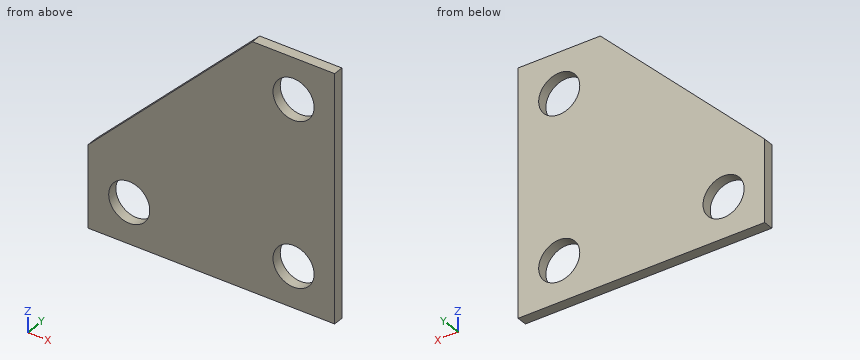
Autodesk Inventor part; units mm, degrees
ref_plane "YZ Plane" through (0, 0, 0) normal (1, 0, 0) x (0, 1, 0)
ref_plane "XZ Plane" through (0, 0, 0) normal (0, 1, 0) x (-1, 0, 0)
ref_plane "XY Plane" through (0, 0, 0) normal (0, 0, 1) x (1, 0, 0)
sketch "Sketch1" plane through (0, 0, 0) normal (0, 1, 0) x (-1, 0, 0)
  line L0 (0, 0) -> (76.2, 0)
  line L1 (76.2, 0) -> (76.2, 25.4)
  line L2 (25.4, 76.2) -> (0, 76.2)
  line L3 (0, 76.2) -> (0, 0)
  line L4 (76.2, 25.4) -> (25.4, 76.2)
  circle A0 centre (63.5, 12.7) radius 6.35
  circle A1 centre (12.7, 63.5) radius 6.35
  circle A2 centre (12.7, 12.7) radius 6.35
  point P0 (76.2, 76.2)
  dimension "d0" = 76.2
  dimension "d1" = 76.2
  dimension "d2" = 50.8
  dimension "d3" = 50.8
  dimension "d4" = 12.7
  dimension "d5" = 12.7
  dimension "d6" = 12.7
  dimension "d7" = 12.7
  dimension "d8" = 50.8
  dimension "d9" = 50.8
  dimension "d10" = 12.7
  dimension "d11" = 12.7
  dimension "d12" = 12.7
extrude "Extrusion1" add sketch "Sketch1" along normal blind 3.175
equation "\"d0\" = d1"
properties part number "3 inch gusset plate"
For this review, take the finished solid that the model builds, in its own axes (mm). Round coordinates to 2 decimals unless told otherwise and drop trailing zeros. Write each loop counter-clockwise with the first axis right and the second up, starting at its lowest first coordinate (ties: lowest second). Pieces come first, ordered by that corner, then holes. Notation, with made-up numbers: (-3.5, -34.75) - (21.5, -34.75) arc R23 ccw to (21.5, -1.75) - close; hole circle Ø1 at (4, 37.25). An arc over 180 degrees is marked (long way). Answer as CSV lines item,"result". Start each with the question number.
(1) Add section B-B, the plane y = 1.05. State the section outline as (x, z) points.
(2) Add section A-A, the plane z = 63.5. State the section outline as (x, y) points (3 decimals).
(3) Add section C-C, the plane x = -12.7. State the section outline as (y, z) points (3 decimals), plus the area to 3 significant figures.
(4) Add section D-D, the plane z = 12.7. State the section outline as (x, y) points (3 decimals), plus the area to 3 significant figures.
(5) For line 1 (Z direction, x = -12.7, y = 1.4); line 2 (Z direction, x = -18.5, y = 0.4); line 3 (X direction, y = 2.95, z = 7), list the stretches that pass through material, from the lowest coordinate up.
(6) For pin 1 (14.5 mm diameter, centred on x = -63.5, z = 12.7, fed in from +Y) (3 decimals), flat-tipped, find the tip position at first contact; note if it passes through.
From the geometry:
1,outline,"(-76.2, 0) - (0, 0) - (0, 76.2) - (-25.4, 76.2) - (-76.2, 25.4) - close; hole circle Ø12.7 at (-63.5, 12.7); hole circle Ø12.7 at (-12.7, 12.7); hole circle Ø12.7 at (-12.7, 63.5)"
2,outline,"(-38.1, 0) - (-19.05, 0) - (-19.05, 3.175) - (-38.1, 3.175) - close; (-6.35, 0) - (0, 0) - (0, 3.175) - (-6.35, 3.175) - close"
3,outline,"(0, 0) - (3.175, 0) - (3.175, 6.35) - (0, 6.35) - close; (0, 19.05) - (3.175, 19.05) - (3.175, 57.15) - (0, 57.15) - close; (0, 69.85) - (3.175, 69.85) - (3.175, 76.2) - (0, 76.2) - close"
3,area,"161 mm²"
4,outline,"(-76.2, 0) - (-69.85, 0) - (-69.85, 3.175) - (-76.2, 3.175) - close; (-57.15, 0) - (-19.05, 0) - (-19.05, 3.175) - (-57.15, 3.175) - close; (-6.35, 0) - (0, 0) - (0, 3.175) - (-6.35, 3.175) - close"
4,area,"161 mm²"
5,line 1,"z = 0 to 6.35, 19.05 to 57.15, 69.85 to 76.2"
5,line 2,"z = 0 to 10.11, 15.29 to 60.91, 66.09 to 76.2"
5,line 3,"x = -76.2 to -66.3, -60.7 to -15.5, -9.9 to 0"
6,pin 1,"stops at y = 3.175"
